from build123d import *

# Parameters (mm, degrees)
BOSS_EXTRUDE1_DEPTH = 4.7625
SKETCH3_W           = 82.55
SKETCH3_H           = 69.85
BOSS_EXTRUDE2_DEPTH = 1.905
SKETCH4_R           = 1.5875
CUT_EXTRUDE1_DEPTH  = 71.351665255


with BuildPart() as part:
    # Sketch1 → Boss-Extrude1 (new body)
    with BuildSketch(Plane(origin=(0, 0, 0), x_dir=(1, 0, 0), z_dir=(0, 1, 0))):
        with BuildLine():
            Line((-46.283113208, 21.781698113), (8.326886792, 21.781698113))
            ThreePointArc((8.326886792, 21.781698113), (10.571950823, 20.851762143), (11.501886792, 18.606698113))
            Line((11.501886792, 18.606698113), (11.501886792, -20.763301887))
            ThreePointArc((11.501886792, -20.763301887), (10.571950823, -23.008365917), (8.326886792, -23.938301887))
            Line((8.326886792, -23.938301887), (-46.283113208, -23.938301887))
            ThreePointArc((-46.283113208, -23.938301887), (-48.528177238, -23.008365917), (-49.458113208, -20.763301887))
            Line((-49.458113208, -20.763301887), (-49.458113208, 18.606698113))
            ThreePointArc((-49.458113208, 18.606698113), (-48.528177238, 20.851762143), (-46.283113208, 21.781698113))
        make_face()
    extrude(amount=BOSS_EXTRUDE1_DEPTH)

    # Sketch3 → Boss-Extrude2 (add)
    with BuildSketch(Plane.XZ):
        with Locations((-18.978113208, 1.078301887)):
            Rectangle(SKETCH3_W, SKETCH3_H)
    extrude(amount=BOSS_EXTRUDE2_DEPTH)

    # Sketch4 → Cut-Extrude1 (cut, through all)
    with BuildSketch(Plane(origin=(0, 0, 0), x_dir=(1, 0, 0), z_dir=(0, 1, 0))):
        with Locations(Location((-53.903113208, 27.496698113, 0), (0, 0, 270))):
            Circle(SKETCH4_R)
        with Locations(Location((15.946886792, 27.496698113, 0), (0, 0, 270))):
            Circle(SKETCH4_R)
        with Locations(Location((15.946886792, -29.653301887, 0), (0, 0, 270))):
            Circle(SKETCH4_R)
        with Locations(Location((-53.903113208, -29.653301887, 0), (0, 0, 270))):
            Circle(SKETCH4_R)
    extrude(amount=-CUT_EXTRUDE1_DEPTH, mode=Mode.SUBTRACT)


solid = part.part
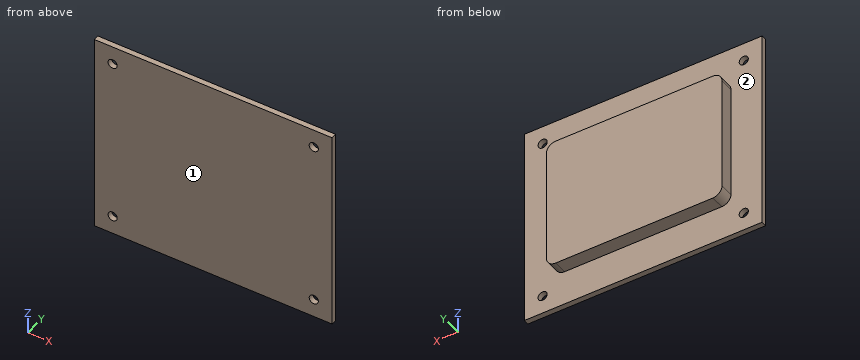
Read the model definition and answer for the solid it produces. Units are mm, in the model's axes. Face numbers are marked on the shaded views. A direction names the side the tool comes from. Round coordinates to 2 decimals unless told otherwise and drop trailing zeros. Loops run counter-clockwise (first coordinate to the right, second up) from the corner with the lowest first, then second, coordinate; pieces in that order, holes last.
Q1. Section B-B on y = 2.5 is taken. Write down the section's boundary in (x, z) (3 decimals).
Q2. Which of the six approach directions +Z, -Z, +X, -X, +Y, -Y give full straight-line access (tool end or side, diameter ignored) to the marked faces 1 and 2?
Q3. Section A-A on z = -14 is taken. Write down the section's boundary in (x, y) (1 decimal).
Q4. Each of these flat-tipped pins is pushed along its axis until it touches: pin 1 (4 mm diameter, centred on y = 2.5, z = -6, fed in from +X); pin 2 (4 mm diameter, centred on x = -23, y = 3.5, fed in from +Z); pin 3 (1 mm diameter, centred on y = 1.5, z = -18.5, fed in from -X). Where does it stop, or does it pass through?
Q5. Consider probe 1 along X at (y, z) = (2.75, -4.5); probe 2 along Y at (x, z) = (-23.5, 31) (3 decimals); probe 3 along Z at (x, y) = (-15, 3.5). Determine where each line is inside the solid, lowest interval first.
Output:
1. outline: (-49.458, -18.607) arc R3.175 ccw to (-46.283, -21.782) - (8.327, -21.782) arc R3.175 ccw to (11.502, -18.607) - (11.502, 20.763) arc R3.175 ccw to (8.327, 23.938) - (-46.283, 23.938) arc R3.175 ccw to (-49.458, 20.763) - close
2. face 1: +Z, -Z, +X, -X, -Y
2. face 2: +Y
3. outline: (-60.3, -1.9) - (22.3, -1.9) - (22.3, 0) - (11.5, 0) - (11.5, 4.8) - (-49.5, 4.8) - (-49.5, 0) - (-60.3, 0) - close
4. pin 1: stops at x = 11.5
4. pin 2: stops at z = 23.94
4. pin 3: stops at x = -49.46
5. probe 1: x = -49.46 to 11.5
5. probe 2: y = -1.905 to 0
5. probe 3: z = -21.78 to 23.94
